```python
from build123d import *

# Parameters (mm, degrees)
BOSS_EXTRUDE1_DEPTH = 5.5
CAVITY1_START       = 134.5
CAVITY1_OUTLINE_W   = 6.666666666
CAVITY1_OUTLINE_H   = 5.5
CAVITY1_DEPTH       = 5.5
SKETCH2_W           = 6.666666667
SKETCH2_H           = 5.1
BOSS_EXTRUDE2_DEPTH = 5.5


# Read off the part's stored shape, not the designer's step: Cavity1
with BuildPart() as part:
    # Sketch1 → Boss-Extrude1 (new body)
    with BuildSketch(Plane.XY):
        Polygon((0, 120), (0, 150), (20, 150), (20, 0), (0, 0), (0, 30), (-5.5, 30), (-5.5, 60), (0, 60), (0, 90), (-5.5, 90), (-5.5, 120), align=None)
    extrude(amount=BOSS_EXTRUDE1_DEPTH)

    # Cavity1 outline → Cavity1 (cut)
    with BuildSketch(Plane(origin=(0, 0, 0), x_dir=(1, 0, 0), z_dir=(0, 1, 0)).offset(CAVITY1_START)):
        with Locations((10, -2.75)):
            Rectangle(CAVITY1_OUTLINE_W, CAVITY1_OUTLINE_H)
    extrude(amount=CAVITY1_DEPTH, mode=Mode.SUBTRACT)

    # Sketch2 → Boss-Extrude2 (add)
    with BuildSketch(Plane.XY.offset(5.5)):
        with Locations((3.333333334, -2.55)):
            Rectangle(SKETCH2_W, SKETCH2_H)
        with Locations((16.666666666, -2.55)):
            Rectangle(SKETCH2_W, SKETCH2_H)
    extrude(amount=-BOSS_EXTRUDE2_DEPTH)


solid = part.part
```
The model under review builds one solid part; all positions refer to its coordinate system, in mm. A direction names the side the tool comes from. Round coordinates to 2 decimals unless told otherwise and drop trailing zeros. Loops run counter-clockwise (first coordinate to the right, second up) from the corner with the lowest first, then second, coordinate; pieces in that order, holes last. Notation, with made-up numbers: (19.25, -10) - (24.25, -10) arc R12 ccw to (24.25, 0) - close; hole circle Ø4 at (52, 51.5). An arc over 180 degrees is marked (long way). Use a Markdown table: item, result. Add a question column.
Q1. Machinability: for faces 4 (the face through (6.667, 137, 3)), 5 (the face through (0, 12, 3)), 6 (the face through (-3, 60, 3)), 7 (the face through (10, 0, 3)), which of the approach directions +Z, -Z, +X, -X, +Y, -Y give a long, thin tool a straight path to every point of the face, cutting with its end or side? Answer none if there is none.
Q2. Insertion check: pin 1 Ø1.6 at (y, z) = (10, 4) entering from -X. The pin has a flat end and moves straight along its axis. Give the tip position at first contact, or say it passes through.
Q3. Add section B-B (z = 1.9). State the section outline as (x, y) points.
Q4. The part is to be moulded in two halves that separate along X. For faces 1 (the face through (0, 135, 3)), 2 (the face through (13.333, 137, 3)), 3 (the face through (-3, 120, 3)), say which applies: pulls with the +X half, pulls with the -X half, needs draft (parallel to the pull), parting line crosses it, or undercut.
Q5. Add section C-C (y = 22). State the section outline as (x, z) points.
Q6. For probe 1 along X at (y, z) = (137, 5.2); probe 2 along Y at (x, z) = (-3.5, 1.5); probe 3 along X at (y, z) = (69.5, 0.5), list the stretches that pass through material, from the lowest coordinate up.
Q7. Add section A-A (x = -2). State the section outline as (y, z) points.
Q8. Add section D-D (x = 9.25). State the section outline as (y, z) points.
Worked answers:
| question | item | result |
|---|---|---|
| 1 | face 4 | +Z, -Z |
| 1 | face 5 | +Z, -Z, -X, -Y |
| 1 | face 6 | +Z, -Z, -X |
| 1 | face 7 | +Z, -Z, -Y |
| 2 | pin 1 | x = 0 |
| 3 | outline | (-5.5, 30) - (0, 30) - (0, -5.1) - (6.67, -5.1) - (6.67, 0) - (13.33, 0) - (13.33, -5.1) - (20, -5.1) - (20, 150) - (0, 150) - (0, 120) - (-5.5, 120) - (-5.5, 90) - (0, 90) - (0, 60) - (-5.5, 60) - close; hole (6.67, 134.5) - (13.33, 134.5) - (13.33, 140) - (6.67, 140) - close |
| 4 | face 1 | pulls with the -X half |
| 4 | face 2 | undercut |
| 4 | face 3 | needs draft |
| 5 | outline | (0, 0) - (20, 0) - (20, 5.5) - (0, 5.5) - close |
| 6 | probe 1 | 0 to 6.67, 13.33 to 20 |
| 6 | probe 2 | 30 to 60, 90 to 120 |
| 6 | probe 3 | 0 to 20 |
| 7 | outline | (30, 0) - (60, 0) - (60, 5.5) - (30, 5.5) - close; (90, 0) - (120, 0) - (120, 5.5) - (90, 5.5) - close |
| 8 | outline | (0, 0) - (134.5, 0) - (134.5, 5.5) - (0, 5.5) - close; (140, 0) - (150, 0) - (150, 5.5) - (140, 5.5) - close |
